from build123d import *

# Parameters (mm, degrees)
SKETCH_W        = 74
SKETCH_H        = 24
PAD_DEPTH       = 20
SKETCH001_W     = 67
SKETCH001_H     = 18
POCKET_DEPTH    = 18
SKETCH002_R     = 0.75
POCKET001_DEPTH = 2
SKETCH003_W     = 3
SKETCH003_H     = 9
POCKET002_DEPTH = 0.4


with BuildPart() as part:
    # Sketch → Pad (new body)
    with BuildSketch(Plane.XY):
        with Locations((37, -12)):
            Rectangle(SKETCH_W, SKETCH_H)
    extrude(amount=PAD_DEPTH)

    # Sketch001 (on Face6 of Pad) → Pocket (cut)
    with BuildSketch(Plane.XY.offset(20)):
        with Locations((36.5, -12)):
            Rectangle(SKETCH001_W, SKETCH001_H)
    extrude(amount=-POCKET_DEPTH, mode=Mode.SUBTRACT)

    # Sketch002 (on Face11 of Pocket) → Pocket001 (cut)
    with BuildSketch(Plane.XY.offset(2)):
        with Locations((3.5, -11)):
            Circle(SKETCH002_R)
        with Locations((69.5, -11)):
            Circle(SKETCH002_R)
    extrude(amount=-POCKET001_DEPTH, mode=Mode.SUBTRACT)

    # Sketch003 (on Face14 of Pocket001) → Pocket002 (cut)
    with BuildSketch(Plane.XY.offset(2)):
        Polygon((9, -9.5), (9, -6.5), (12, -6.5), (12, -9.5), (15, -9.5), (15, -12.5), (12, -12.5), (12, -15.5), (9, -15.5), (9, -12.5), (6, -12.5), (6, -9.5), align=None)
        with Locations((65.5, -11)):
            Rectangle(SKETCH003_W, SKETCH003_H)
    extrude(amount=-POCKET002_DEPTH, mode=Mode.SUBTRACT)


solid = part.part
Geometry check sheet. Reference: the model listing, model coordinates, mm. A direction names the side the tool comes from. Round coordinates to 2 decimals unless told otherwise and drop trailing zeros. Order: outer loops, then holes, each group sorted by start corner. A loop starts at its lowest first (then second) coordinate and runs counter-clockwise, first axis right, second up. Notation, with made-up numbers: (50, 27) -> (98, 27) arc R13 cw to (98, 33) -> close; hole circle Ø1 at (75.5, 74). An arc over 180 degrees is marked (long way). Use one line per item in the form item = value.
1. Cross-section at B-B, the plane y = -13.75. Enter the section's corners in (x, z).
Working result:
outline = (0, 0) -> (74, 0) -> (74, 20) -> (70, 20) -> (70, 2) -> (67, 2) -> (67, 1.6) -> (64, 1.6) -> (64, 2) -> (12, 2) -> (12, 1.6) -> (9, 1.6) -> (9, 2) -> (3, 2) -> (3, 20) -> (0, 20) -> close
2. Cross-section at A-A, the plane z = 14.5. Enter the section's corners in (x, y), plus the area to 3 significant figures.
Working result:
outline = (0, -24) -> (74, -24) -> (74, 0) -> (0, 0) -> close; hole (3, -21) -> (70, -21) -> (70, -3) -> (3, -3) -> close
area = 570 mm^2
3. Cross-section at C-C, the plane x = 58. Enter the section's corners in (y, z), plus the area to 3 significant figures.
Working result:
outline = (-24, 0) -> (0, 0) -> (0, 20) -> (-3, 20) -> (-3, 2) -> (-21, 2) -> (-21, 20) -> (-24, 20) -> close
area = 156 mm^2
4. Mould release check, pull along Y, two halves, no side actions. Record for faces 4 (the face through (65, -11, 1.6)), 5 (the face through (34, -22, 20)), 6 (the face through (36, -24, 10)), 7 (the face through (3, -12, 11)): pulls with the +Y half, pulls with the -Y half, needs draft (parallel to the pull), parting line crosses it, or undercut.
Working result:
face_4 = undercut
face_5 = needs draft
face_6 = pulls with the -Y half
face_7 = undercut
5. Scan lines: line 1 along Y through (x, z) = (25.5, 3.75); line 2 along X through (y, z) = (-8, 8.5); line 3 along Y through (x, z) = (3.5, 0.5). Record each from-to range of solid material in increasing order. Write a range as from..to.
Working result:
line_1 = -24..-21, -3..0
line_2 = 0..3, 70..74
line_3 = -24..-11.75, -10.25..0
6. Set-up check for faces 1 (the face through (68.75, -10.97, 1.01)), 2 (the face through (0, -12, 10)), 3 (the face through (36, -3, 11)): record each of +Z, -Z, +X, -X, +Y, -Y from which the full face is reachable in a straight line by a thin tool's end or side.
Working result:
face_1 = -Z
face_2 = +Z, -Z, -X, +Y, -Y
face_3 = +Z
7. Cross-section at D-D, the plane y = -4. Enter the section's corners in (x, z), plus the area to 3 significant figures.
Working result:
outline = (0, 0) -> (74, 0) -> (74, 20) -> (70, 20) -> (70, 2) -> (3, 2) -> (3, 20) -> (0, 20) -> close
area = 274 mm^2
8. Go/stop test with a flat-tipped pin: pin 1 (2.5 mm diameter, centred on x = 66, y = -12.5, fed in from +Z). Record where the tip stops, or that it passes through.
Working result:
pin_1 = 2
